```python
from build123d import *

# Parameters (mm, degrees)
BOSS_EXTRUDE8_DEPTH      = 12
SKETCH2_W                = 10
SKETCH2_H                = 9
BOSS_EXTRUDE9_DEPTH      = 1
BOSS_EXTRUDE9_DEPTH_BACK = 5.8
SKETCH3_R                = 1.5
CUT_EXTRUDE1_DEPTH       = 10
SKETCH4_W                = 8
SKETCH4_H                = 4
BOSS_EXTRUDE10_DEPTH     = 12
SKETCH5_R                = 1.5
CUT_EXTRUDE2_DEPTH       = 12
FILLET2_R                = 3
FILLET3_R                = 3
FILLET4_R                = 3
FILLET5_R                = 3
FILLET6_R                = 3
SKETCH6_R                = 1.5
CUT_EXTRUDE4_DEPTH       = 20
SKETCH7_R                = 1.5
CUT_EXTRUDE5_DEPTH       = 30


with BuildPart() as part:
    # Sketch1 → Boss-Extrude8 (new body)
    with BuildSketch(Plane.XY):
        with BuildLine():
            Line((25, 0), (19.5, 0))
            ThreePointArc((19.5, 0), (0, -19.5), (-19.5, 0))
            Line((-19.5, 0), (-25, 0))
            ThreePointArc((-25, 0), (-20.916500663, -13.693063938), (-10, -22.912878475))
            ThreePointArc((-10, -22.912878475), (0, -25), (10, -22.912878475))
            ThreePointArc((10, -22.912878475), (20.916500663, -13.693063938), (25, 0))
        make_face()
        with BuildLine():
            Line((10, -62.912878475), (10, -22.912878475))
            ThreePointArc((10, -22.912878475), (0, -25), (-10, -22.912878475))
            Line((-10, -22.912878475), (-10, -62.912878475))
            Line((-10, -62.912878475), (10, -62.912878475))
        make_face()
    extrude(amount=BOSS_EXTRUDE8_DEPTH)

    # Sketch2 → Boss-Extrude9 (add, two sides)
    with BuildSketch(Plane(origin=(0, 0, 0), x_dir=(-1, 0, 0), z_dir=(0, 0, -1))) as boss_extrude9_sk:
        with Locations((27.5, 0)):
            Rectangle(SKETCH2_W, SKETCH2_H)
    extrude(amount=BOSS_EXTRUDE9_DEPTH)
    extrude(boss_extrude9_sk.sketch, amount=-BOSS_EXTRUDE9_DEPTH_BACK)

    # Sketch3 → Cut-Extrude1 (cut)
    with BuildSketch(Plane(origin=(0, 0, -1), x_dir=(-1, 0, 0), z_dir=(0, 0, -1))):
        with Locations((28.5, 0.5)):
            Circle(SKETCH3_R)
    extrude(amount=-CUT_EXTRUDE1_DEPTH, mode=Mode.SUBTRACT)

    # Sketch4 → Boss-Extrude10 (add)
    with BuildSketch(Plane(origin=(0, 0, 0), x_dir=(-1, 0, 0), z_dir=(0, 0, -1))):
        with Locations((-27.5, -2)):
            Rectangle(SKETCH4_W, SKETCH4_H)
    extrude(amount=-BOSS_EXTRUDE10_DEPTH)

    # Sketch5 → Cut-Extrude2 (cut)
    with BuildSketch(Plane.XZ.offset(4)):
        with Locations((28.177925359, 6)):
            Circle(SKETCH5_R)
    extrude(amount=-CUT_EXTRUDE2_DEPTH, mode=Mode.SUBTRACT)

    # Fillet2
    fillet2_edges = [part.edges().sort_by_distance(p)[0] for p in [
        (-32.5, -4.5, 2.4),
    ]]
    fillet(fillet2_edges, radius=FILLET2_R)

    # Fillet3
    fillet3_edges = [part.edges().sort_by_distance(p)[0] for p in [
        (-32.5, 4.5, 2.4),
    ]]
    fillet(fillet3_edges, radius=FILLET3_R)

    # Fillet4
    fillet4_edges = [part.edges().sort_by_distance(p)[0] for p in [
        (-22.5, 4.5, 2.4),
    ]]
    fillet(fillet4_edges, radius=FILLET4_R)

    # Fillet5
    fillet5_edges = [part.edges().sort_by_distance(p)[0] for p in [
        (31.5, -2, 0),
    ]]
    fillet(fillet5_edges, radius=FILLET5_R)

    # Fillet6
    fillet6_edges = [part.edges().sort_by_distance(p)[0] for p in [
        (31.5, -2, 12),
    ]]
    fillet(fillet6_edges, radius=FILLET6_R)

    # Sketch6 → Cut-Extrude4 (cut)
    with BuildSketch(Plane(origin=(0, 0, 0), x_dir=(-1, 0, 0), z_dir=(0, 0, -1))):
        with Locations((0, -37.912878475)):
            Circle(SKETCH6_R)
        with Locations((0, -52.912878475)):
            Circle(SKETCH6_R)
    extrude(amount=-CUT_EXTRUDE4_DEPTH, mode=Mode.SUBTRACT)

    # Sketch7 → Cut-Extrude5 (cut)
    with BuildSketch(Plane(origin=(10, 0, 0), x_dir=(0, 0, -1), z_dir=(1, 0, 0))):
        with Locations((-6, -45.412878475)):
            Circle(SKETCH7_R)
    extrude(amount=-CUT_EXTRUDE5_DEPTH, mode=Mode.SUBTRACT)


solid = part.part
```
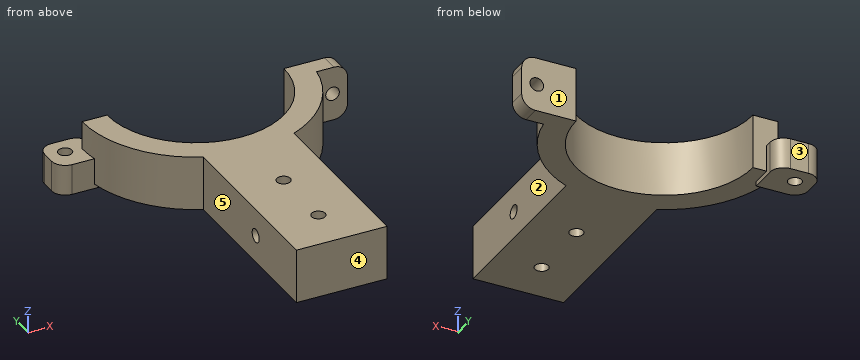
The listing builds one solid part. Answer for the finished solid, in the listing's coordinates (mm). Face numbers are marked on the shaded views. A direction names the side the tool comes from. Give positions to 0.01 mm unless a question says otherwise; leave off trailing zeros. Order: outer loops, then holes, each group sorted by start corner. A loop starts at its lowest first (then second) coordinate and runs counter-clockwise, first axis right, second up. Notation, with made-up numbers: (-19.75, 59) -> (1.25, 59) arc R25 cw to (1.25, 74) -> close; hole circle Ø4 at (53, 15). An arc over 180 degrees is marked (long way). Answer as a JSON object with one key per item and string values. Group by question number.
Item 1: The part is cut by section A-A on x = -28.5. Write down the section's boundary in (y, z).
Item 2: A tool of negligible diameter and unlimited length cuts with its end or side. For the marked faces 1, 2, 3, 4 and 5, from which of +Z, -Z, +X, -X, +Y, -Y can it reach the whole face along a straight path? Write none if from no direction.
Item 3: The part is cut by section D-D on z = 1.5. Write down the section's boundary in (x, y).
Item 4: Flat-ended cylindrical pins translate along their axes: pin 1 (5 mm diameter, centred on x = 0, y = -52.91, fed in from -Z); pin 2 (1.8 mm diameter, centred on x = 0, y = -37.91, fed in from +Z); pin 3 (5 mm diameter, centred on x = 28.18, z = 6, fed in from -Y); pin 4 (2 mm diameter, centred on x = -14.5, z = 9, fed in from -Y). Find the tip coordinate at first contact, or state that the pin passes through.
Item 5: The part is cut by section B-B on x = 0. Write down the section's boundary in (y, z).
Item 6: The part is cut by section C-C on y = -2.5. Write down the section's boundary in (x, z).
Item 7: Consider L1, parallel to Y at x = 0, z = 3.5; L2, parallel to X at y = -53, z = 9.25; L3, parallel to Y at x = -28.5, z = 1.5. Determine where each line is inside the solid, lowest interval first. Write a range as from..to.
Result set:
{
 "1": {"outline": "(-4.5, -1) -> (-1, -1) -> (-1, 5.8) -> (-4.5, 5.8) -> close; (2, -1) -> (4.5, -1) -> (4.5, 5.8) -> (2, 5.8) -> close"},
 "2": {"face 1": "+Z, -Z, +X, +Y", "face 2": "+Z, -Z, +X, -Y", "face 3": "+Z, -Z, +X, -X, +Y", "face 4": "+Z, -Z, +X, -X, -Y", "face 5": "+Z, -Z, -X, -Y"},
 "3": {"outline": "(-32.5, -1.5) arc R3 ccw to (-29.5, -4.5) -> (-24.59, -4.5) arc R25 ccw to (-10, -22.91) -> (-10, -62.91) -> (10, -62.91) -> (10, -22.91) arc R25 ccw to (24.68, -4) -> (31.1, -4) -> (31.1, 0) -> (19.5, 0) arc R19.5 cw to (-19.5, 0) -> (-22.5, 0) -> (-22.5, 1.5) arc R3 ccw to (-25.5, 4.5) -> (-29.5, 4.5) arc R3 ccw to (-32.5, 1.5) -> close; hole circle Ø3 at (-28.5, 0.5); hole circle Ø3 at (0, -52.91); hole circle Ø3 at (0, -37.91)"},
 "4": {"pin 1": "z = 0", "pin 2": "through", "pin 3": "y = -4", "pin 4": "y = -21.04"},
 "5": {"outline": "(-62.91, 0) -> (-54.41, 0) -> (-54.41, 12) -> (-62.91, 12) -> close; (-51.41, 0) -> (-39.41, 0) -> (-39.41, 12) -> (-51.41, 12) -> close; (-36.41, 0) -> (-19.5, 0) -> (-19.5, 12) -> (-36.41, 12) -> close; hole circle Ø3 at (-45.41, 6)"},
 "6": {"outline": "(-32.33, -1) -> (-22.5, -1) -> (-22.5, 0) -> (-19.34, 0) -> (-19.34, 12) -> (-24.87, 12) -> (-24.87, 5.8) -> (-32.33, 5.8) -> close; (19.34, 0) -> (28.5, 0) arc R3 ccw to (31.5, 3) -> (31.5, 9) arc R3 ccw to (28.5, 12) -> (19.34, 12) -> close; hole circle Ø3 at (28.18, 6)"},
 "7": {"L1": "-62.91..-54.41, -51.41..-39.41, -36.41..-19.5", "L2": "-10..-1.5, 1.5..10", "L3": "-4.5..-1, 2..4.5"}
}
